Geometry check sheet. Reference: the model listing, model coordinates, mm. Face numbers are marked on the shaded views. A direction names the side the tool comes from. Give positions to 0.01 mm unless a question says otherwise; leave off trailing zeros. Order: outer loops, then holes, each group sorted by start corner. A loop starts at its lowest first (then second) coordinate and runs counter-clockwise, first axis right, second up.
from build123d import *

# Parameters (mm, degrees)
CUT_EXTRUDE1_DEPTH  = 15.35
CIRPATTERN1_COUNT   = 17
SKETCH3_R           = 3.5
BOSS_EXTRUDE1_DEPTH = 20


with BuildPart() as part:
    # Sketch1 → Revolve1 (revolve)
    with BuildSketch(Plane(origin=(0, 0, 0), x_dir=(0, 0, -1), z_dir=(1, 0, 0))):
        Polygon((0, 0), (0, 57), (5, 57), (5, 25.000000038), (14.35, 25.000000038), (14.35, 0), align=None)
    revolve(axis=Axis((0, 0, -14.35), (0, 0, 1)))

    # Sketch2 → Cut-Extrude1 (cut, through all)
    with BuildSketch(Plane(origin=(0, 0, -14.35), x_dir=(-1, 0, 0), z_dir=(0, 0, -1))):
        with BuildLine():
            Line((0, 0), (0, 18.8))
            ThreePointArc((0, 18.8), (1.734645158, 18.719802514), (3.454490935, 18.479894274))
            Line((3.454490935, 18.479894274), (3.685673166, 16.390723392))
            ThreePointArc((3.685673166, 16.390723392), (4.597538233, 16.158670805), (5.494981484, 15.875930791))
            Line((5.494981484, 15.875930791), (6.791343324, 17.530477913))
            Line((6.791343324, 17.530477913), (0, 0))
        make_face()
    cut_extrude1 = extrude(amount=-CUT_EXTRUDE1_DEPTH, mode=Mode.SUBTRACT)

    # CirPattern1: Cut-Extrude1 ×17 about axis
    cirpattern1_axis = Axis((0, 0, 0), (0, 0, 1))
    for i in range(1, CIRPATTERN1_COUNT):
        add(cut_extrude1.rotate(cirpattern1_axis, i * 360 / CIRPATTERN1_COUNT), mode=Mode.SUBTRACT)

    # Sketch3 → Boss-Extrude1 (add)
    with BuildSketch(Plane.XY):
        with Locations((0, 42)):
            Circle(SKETCH3_R)
        with Locations((29.69848481, 29.69848481)):
            Circle(SKETCH3_R)
        with Locations((42, 0)):
            Circle(SKETCH3_R)
        with Locations((29.69848481, -29.69848481)):
            Circle(SKETCH3_R)
        with Locations((0, -42)):
            Circle(SKETCH3_R)
        with Locations((-29.69848481, -29.69848481)):
            Circle(SKETCH3_R)
        with Locations((-42, 0)):
            Circle(SKETCH3_R)
        with Locations((-29.69848481, 29.69848481)):
            Circle(SKETCH3_R)
    extrude(amount=BOSS_EXTRUDE1_DEPTH)


solid = part.part
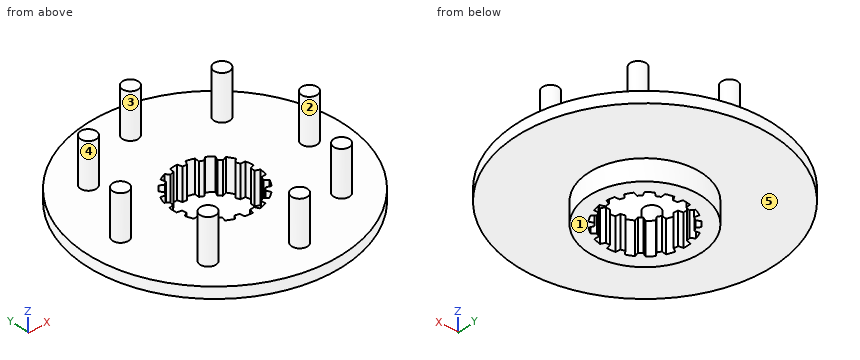
Item 1: Sectioned sample at B-B (y = 42). Enter the section's corners in (x, z).
Reported:
outline: (-38.54, -5) - (38.54, -5) - (38.54, 0) - (3.5, 0) - (3.5, 20) - (-3.5, 20) - (-3.5, 0) - (-38.54, 0) - close
Item 2: Draft check along X on the marked faces 1, 2 and 3. Enter one of: released by +X, released by -X, zero draft, split by the parting line, or undercut.
Reported:
face 1: zero draft
face 2: undercut
face 3: split by the parting line
Item 3: Sectioned sample at C-C (x = 31). Enter the section's corners in (y, z).
Reported:
outline: (-47.83, -5) - (47.83, -5) - (47.83, 0) - (32.95, 0) - (32.95, 20) - (26.45, 20) - (26.45, 0) - (-26.45, 0) - (-26.45, 20) - (-32.95, 20) - (-32.95, 0) - (-47.83, 0) - close
Item 4: Scan lines: L1, parallel to Y at x = 12.5, z = -5.5; L2, parallel to Z at x = -51.5, y = -8; L3, parallel to Y at x = -2, z = 18. Record each from-to range of solid material in increasing order.
Reported:
L1: y = -21.65 to -14.04, -13.55 to -11.22, 11.22 to 13.55, 14.04 to 21.65
L2: z = -5 to 0
L3: y = -44.87 to -39.13, 39.13 to 44.87
Item 5: Sectioned sample at A-A (z = 15). Enter the section's corners in (x, y).
Reported:
outline: circle Ø7 at (-42, 0); circle Ø7 at (-29.7, -29.7); circle Ø7 at (-29.7, 29.7); circle Ø7 at (0, -42); circle Ø7 at (0, 42); circle Ø7 at (29.7, -29.7); circle Ø7 at (29.7, 29.7); circle Ø7 at (42, 0)
Item 6: Set-up check for the marked faces 4 and 5: record each of +Z, -Z, +X, -X, +Y, -Y from which the full face is reachable in a straight line by a thin tool's end or side.
Reported:
face 4: +Z
face 5: -Z
Item 7: Gauge pin test, flat ends, axial feed: pin 1 (4 mm diameter, centred on x = 0.5, y = 41, fed in from -Z); pin 2 (3 mm diameter, centred on y = 7.5, z = 1, fed in from +X); pin 3 (5 mm diameter, centred on x = 10.5, z = -9.5, fed in from +Y). Record the tip position at first contact, or that the pin passes through.
Reported:
pin 1: stops at z = -5
pin 2: stops at x = 56.64
pin 3: stops at y = 23.69
